```python
from build123d import *

# Parameters (mm, degrees)
F0_W     = 2
F0_H     = 79
F0_R     = 1.5
F1_DEPTH = 25


with BuildPart() as f1:
    # F0 (on Top) → F1 (new body)
    with BuildSketch(Plane.XY):
        with BuildLine():
            Line((116.5, 8), (0, 8))
            ThreePointArc((0, 8), (-7.977735, -0.596449), (1.189577, -7.911062))
            Line((1.189577, -7.911062), (31.5, -3.353319))
            Line((31.5, -3.353319), (90.5, -10.871761))
            Line((90.5, -10.871761), (90.5, -89))
            ThreePointArc((90.5, -89), (94.307612, -98.192388), (103.5, -102))
            ThreePointArc((103.5, -102), (112.692388, -98.192388), (116.5, -89))
            Line((116.5, -89), (116.5, 8))
        make_face()
        with Locations((104, -49.5)):
            Rectangle(F0_W, F0_H, mode=Mode.SUBTRACT)
        Circle(F0_R, mode=Mode.SUBTRACT)
        with Locations((63, 0)):
            Circle(F0_R, mode=Mode.SUBTRACT)
    extrude(amount=F1_DEPTH)


solid = f1.part
```
Geometry check sheet. Reference: the model listing, model coordinates, mm. A direction names the side the tool comes from. Give positions to 0.01 mm unless a question says otherwise; leave off trailing zeros. Loops run counter-clockwise (first coordinate to the right, second up) from the corner with the lowest first, then second, coordinate; pieces in that order, holes last. Notation, with made-up numbers: M 64,-24.5 L 79,-24.5 A34 cw 79,7.5 Z; hole C -8.5,81.25 d2. An arc over 180 degrees is marked long. Answer as CSV lines item,"result".
Item 1: Release check for a two-part mould opening along Y. For faces 1 (the flat face through (91, -30, 0)), 2 (the cylindrical face through (-8, 0, 12)), 3 (the flat face through (105, -50, 12)) record: pulls with the +Y half, pulls with the -Y half, needs draft (parallel to the pull), parting line crosses it, or undercut.
Values:
face 1,"needs draft"
face 2,"parting line crosses it"
face 3,"undercut"
Item 2: Material ranges on line 1 (X direction, y = -42, z = 14.5); line 2 (Y direction, x = 0, z = 10.75); line 3 (Y direction, x = 63, z = 9), recorded low to high.
Values:
line 1,"x = 90.5 to 103, 105 to 116.5"
line 2,"y = -8 to -1.5, 1.5 to 8"
line 3,"y = -7.37 to -1.5, 1.5 to 8"
Item 3: Cross-section at A-A on y = -64. Record the cut outline in (x, z), and give its area (3 significant figures).
Values:
outline,"M 90.5,0 L 103,0 L 103,25 L 90.5,25 Z; M 105,0 L 116.5,0 L 116.5,25 L 105,25 Z"
area,"600 mm²"
Item 4: Cross-section at D-D on y = 0. Record the cut outline in (x, z), and give its area (3 significant figures).
Values:
outline,"M -8,0 L -1.5,0 L -1.5,25 L -8,25 Z; M 1.5,0 L 61.5,0 L 61.5,25 L 1.5,25 Z; M 64.5,0 L 116.5,0 L 116.5,25 L 64.5,25 Z"
area,"2,960 mm²"
Item 5: Depth check by flat-ended pin: P1, Ø6, axis at x = 100, z = 22, coming from the -Y side; P2, Ø1, axis at x = 94.5, y = -3, coming from the -Z side; P3, Ø2, axis at x = 33.5, z = 8, coming from the -Y side; P4, Ø12, axis at x = 38.5, z = 10, coming from the -Y side. Enter the tip coordinate at first touch or a pass-through.
Values:
P1,"stops at y = -101.99"
P2,"stops at z = 0"
P3,"stops at y = -3.74"
P4,"stops at y = -5.01"
Item 6: Access from +Z, -Z, +X, -X, +Y, -Y to the whole of each face (thin tool, end or side, straight path). Record for faces 4 (the flat face through (60.59, -7.06, 12.32)), 5 (the flat face through (103, -50, 12)), 6 (the flat face through (90.5, -49, 12)).
Values:
face 4,"+Z, -Z, -Y"
face 5,"+Z, -Z"
face 6,"+Z, -Z, -X, -Y"
Item 7: Cross-section at B-B on z = 8.25. Record the cut outline in (x, y).
Values:
outline,"M 0,8 A8 ccw long 1.19,-7.91 L 31.5,-3.35 L 90.5,-10.87 L 90.5,-89 A13 ccw 103.5,-102 A13 ccw 116.5,-89 L 116.5,8 Z; hole C 0,0 d3; hole C 63,0 d3; hole M 103,-89 L 105,-89 L 105,-10 L 103,-10 Z"
Item 8: Cross-section at C-C on x = 63. Record the cut outline in (y, z), and give its area (3 significant figures).
Values:
outline,"M -7.37,0 L -1.5,0 L -1.5,25 L -7.37,25 Z; M 1.5,0 L 8,0 L 8,25 L 1.5,25 Z"
area,"309 mm²"
